from build123d import *

# Parameters (mm, degrees)
PAD_DEPTH       = 12
POCKET_DEPTH    = 4
SKETCH002_R     = 5.25
PAD001_DEPTH    = 20
SKETCH003_R     = 1.75
POCKET001_DEPTH = 28.001
FILLET_R        = 3
FILLET001_R     = 2
FILLET002_R     = 5


with BuildPart() as part:
    # Sketch001 → Pad (new body)
    with BuildSketch(Plane.XY):
        with BuildLine():
            ThreePointArc((14, 0), (0, 14), (-14, 0))
            Line((-14, 0), (-14, -42))
            ThreePointArc((-14, -42), (0, -56), (14, -42))
            Line((14, -42), (14, 0))
        make_face()
    extrude(amount=PAD_DEPTH)

    # Sketch (on Face6 of Pad) → Pocket (cut)
    with BuildSketch(Plane.XY.offset(12)):
        with BuildLine():
            ThreePointArc((6.309715, -4.5), (0, 7.75), (-6.309715, -4.5))
            Line((-6.309715, -4.5), (-4.245292, -8))
            Line((-4.245292, -8), (-4.245292, -23.7))
            ThreePointArc((-4.245292, -23.7), (0, -27.75), (4.245292, -23.7))
            Line((4.245292, -8), (4.245292, -23.7))
            Line((6.309715, -4.5), (4.245292, -8))
        make_face()
    extrude(amount=-POCKET_DEPTH, mode=Mode.SUBTRACT)

    # Sketch002 (on Face4 of Pocket) → Pad001 (join)
    with BuildSketch(Plane(origin=(0, 0, 0), x_dir=(1, 0, 0), z_dir=(0, 0, -1))):
        with Locations((0, 42)):
            Circle(SKETCH002_R)
    extrude(amount=PAD001_DEPTH)

    # Sketch003 (on Face15 of Pad001) → Pocket001 (cut, through all)
    with BuildSketch(Plane.XY.offset(8)):
        Circle(SKETCH003_R)
        with Locations((0, -23.5)):
            Circle(SKETCH003_R)
    extrude(amount=-POCKET001_DEPTH, mode=Mode.SUBTRACT)

    # Fillet
    fillet_edges = [part.edges().sort_by_distance(p)[0] for p in [
        (-5.25, -42, 0),
    ]]
    fillet(fillet_edges, radius=FILLET_R)

    # Fillet001
    fillet001_edges = [part.edges().sort_by_distance(p)[0] for p in [
        (-14, -21, 0),
        (0, 14, 0),
        (14, -21, 0),
        (0, -56, 0),
    ]]
    fillet(fillet001_edges, radius=FILLET001_R)

    # Fillet002
    fillet002_edges = [part.edges().sort_by_distance(p)[0] for p in [
        (-4.245292, -8, 10),
        (4.245292, -8, 10),
    ]]
    fillet(fillet002_edges, radius=FILLET002_R)


solid = part.part
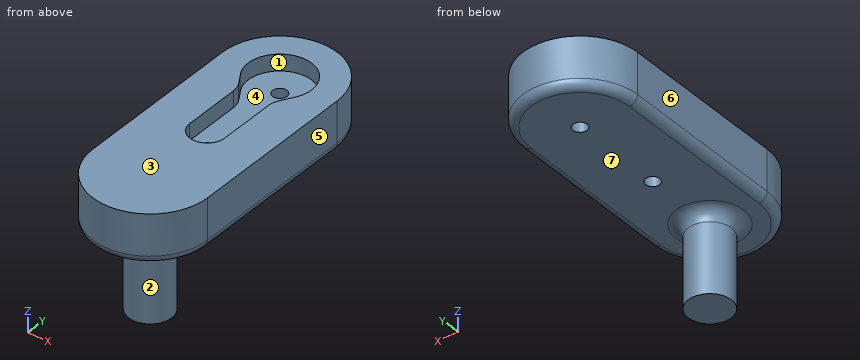
Can you work these out from the model? Positions are in its coordinate system, mm. Face numbers are marked on the shaded views. A direction names the side the tool comes from. Coordinates: 2 decimals unless noted, no trailing zeros. Write each loop counter-clockwise with the first axis right and the second up, starting at its lowest first coordinate (ties: lowest second). Pieces come first, ordered by that corner, then holes. Notation, with made-up numbers: (55, 17.25) - (79, 17.25) arc R6 ccw to (79, 28.25) - close; hole circle Ø3 at (88.25, 64.5). An arc over 180 degrees is marked (long way). Return JSON: item names as keys, results as strings. Group by question number.
Item 1: If we section it at C-C (z = -15.5): Write out the boundary of the cut face in (x, y), then the cut area to 3 significant figures.
Item 2: We'd pull the mould along X, two halves only. Please class the marked faces 4, 5, 6 and 7: pulls with the +X half, pulls with the -X half, needs draft (parallel to the pull), parting line crosses it, or undercut.
Item 3: If we section it at D-D (y = -29.5): Write out the boundary of the cut face in (x, z).
Item 4: Please list where these lines run through material, in increasing order: probe 1 along Y at (x, z) = (0, 5.5); probe 2 along Y at (x, z) = (0, 10.65); probe 3 along X at (y, z) = (0, 11).
Item 5: If we section it at B-B (y = -10.5): Write out the boundary of the cut face in (x, z), then the cut area to 3 significant figures.
Item 6: I'm going to push flat-ended pins straight in: pin 1 Ø5 at (x, z) = (-4, 4.5) entering from -Y; pin 2 Ø8 at (x, z) = (1, -15.5) entering from -Y; pin 3 Ø12.5 at (x, y) = (0, 0) entering from +Z; pin 4 Ø12 at (y, z) = (-27.5, -8) entering from +X. Where does each tip first touch, or does it pass through?
Item 7: Which directions (+Z, -Z, +X, -X, +Y, -Y) give clear straight access to the entire face, cutting with the end or side of a thin tool? Please do the marked faces 1, 2 and 3.
Item 8: If we section it at A-A (x = 0): Write out the boundary of the cut face in (y, z).
Return value:
{
 "1": {"outline": "circle Ø10.5 at (0, -42)", "area": "86.6 mm^2"},
 "2": {"face 4": "undercut", "face 5": "pulls with the +X half", "face 6": "pulls with the -X half", "face 7": "needs draft"},
 "3": {"outline": "(-14, 2) arc R2 ccw to (-12, 0) - (12, 0) arc R2 ccw to (14, 2) - (14, 12) - (-14, 12) - close"},
 "4": {"probe 1": "y = -56 to -25.25, -21.75 to -1.75, 1.75 to 14", "probe 2": "y = -56 to -27.75, 7.75 to 14", "probe 3": "x = -14 to -7.75, 7.75 to 14"},
 "5": {"outline": "(-14, 2) arc R2 ccw to (-12, 0) - (12, 0) arc R2 ccw to (14, 2) - (14, 12) - (4.25, 12) - (4.25, 8) - (-4.25, 8) - (-4.25, 12) - (-14, 12) - close", "area": "300 mm^2"},
 "6": {"pin 1": "stops at y = -55.92", "pin 2": "stops at y = -47.25", "pin 3": "stops at z = 8", "pin 4": "passes through"},
 "7": {"face 1": "+Z", "face 2": "-Z", "face 3": "+Z, +X, -X, +Y, -Y"},
 "8": {"outline": "(-56, 2) arc R2 ccw to (-54, 0) - (-50.25, 0) arc R3 cw to (-47.25, -3) - (-47.25, -20) - (-36.75, -20) - (-36.75, -3) arc R3 cw to (-33.75, 0) - (-25.25, 0) - (-25.25, 8) - (-27.75, 8) - (-27.75, 12) - (-56, 12) - close; (-21.75, 0) - (-1.75, 0) - (-1.75, 8) - (-21.75, 8) - close; (1.75, 0) - (12, 0) arc R2 ccw to (14, 2) - (14, 12) - (7.75, 12) - (7.75, 8) - (1.75, 8) - close"}
}
